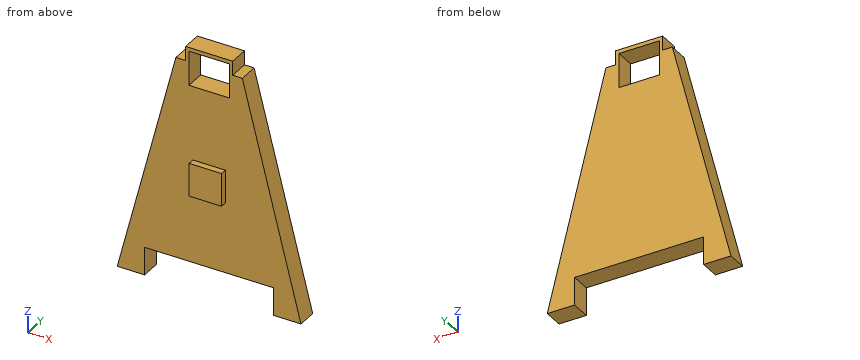
```python
from build123d import *

# Parameters (mm, degrees)
F0_W     = 1.090225624
F0_H     = 7.7231296032
F1_DEPTH = 6.35
F3_DEPTH = 8.39926


with BuildPart() as f1:
    # F0 (on Front) → F1 (new body)
    with BuildSketch(Plane.XZ):
        Polygon((-7.5686656406, 37.2254792051), (-10.668, 37.2254792051), (-29.5124314971, -36.6076258465), (-20.7240314971, -36.6076258465), (-20.7240314971, -27.6487994939), (0, -27.6487994939), (20.7240314971, -27.6487994939), (20.7240314971, -36.6076258465), (29.5124314971, -36.6076258465), (10.668, 37.2254792051), (7.5686656406, 37.2254792051), (7.5686656406, 29.5023496019), (6.4784400165, 29.5023496019), (0, 29.5023496019), (-6.4784400165, 29.5023496019), (-7.5686656406, 29.5023496019), align=None)
        with Locations((-7.0235528285, 33.3639144035)):
            Rectangle(F0_W, F0_H)
        Polygon((-7.5686656406, 41.7925901711), (-7.5686656406, 37.2254792051), (-6.4784400165, 37.2254792051), (-6.4784400165, 40.5764468014), (0, 40.5764468014), (6.4784400165, 40.5764468014), (6.4784400165, 37.2254792051), (7.5686656406, 37.2254792051), (7.5686656406, 41.7925901711), (0, 41.7925901711), align=None)
        with Locations((7.0235528285, 33.3639144035)):
            Rectangle(F0_W, F0_H)
    extrude(amount=F1_DEPTH)

    # F2 (on Front) → F3 (join)
    with BuildSketch(Plane.XZ):
        Polygon((0, 5.6396927685), (-5.2173733711, 5.6396927685), (-5.2173733711, -4.9869618379), (0, -4.9869618379), (5.2173733711, -4.9869618379), (5.2173733711, 5.6396927685), align=None)
    extrude(amount=F3_DEPTH)


solid = f1.part
```
Check sheet for the modelled part. Datum: model origin and axes. Units: mm. Round coordinates to 2 decimals unless told otherwise and drop trailing zeros. Order: outer loops, then holes, each group sorted by start corner. A loop starts at its lowest first (then second) coordinate and runs counter-clockwise, first axis right, second up. Notation, with made-up numbers: M 31,89 L 83,89 A11 ccw 83,97 Z; hole C 31.5,-26 d3. An arc over 180 degrees is marked long. Answer in a Markdown table with one row per item.
(1) Gauge pin test, flat ends, axial feed: pin 1 (12 mm diameter, centred on x = 20, z = 27, fed in from +Y); pin 2 (2 mm diameter, centred on x = -16, y = -3.5, fed in from -Z); pin 3 (3 mm diameter, centred on y = -7, z = 26, fed in from -X); pin 4 (0.9 mm diameter, centred on x = -9, y = -2, fed in from +Z). Record the tip position at first contact, or that the pin passes through.
Findings:
| item | result |
|---|---|
| pin 1 | passes through |
| pin 2 | stops at z = -27.65 |
| pin 3 | stops at x = -13.88 |
| pin 4 | stops at z = 37.23 |
(2) Section check A-A on x = 3. Record the boundary of the cut face in (y, z).
Findings:
| item | result |
|---|---|
| outline | M -8.4,-4.99 L -6.35,-4.99 L -6.35,-27.65 L 0,-27.65 L 0,29.5 L -6.35,29.5 L -6.35,5.64 L -8.4,5.64 Z; M -6.35,40.58 L 0,40.58 L 0,41.79 L -6.35,41.79 Z |
(3) Material ranges on line 1 along Z through (x, y) = (-4, -5.5); line 2 along Y through (x, z) = (2, 15.5); line 3 along Z through (x, y) = (9, -5.5), recorded low to high. Write a range as from..to.
Findings:
| item | result |
|---|---|
| line 1 | z = -27.65..29.5, 40.58..41.79 |
| line 2 | y = -6.35..0 |
| line 3 | z = -27.65..37.23 |
(4) Section check C-C on z = 36. Record the boundary of the cut face in (x, y), plus the area to 3 significant figures.
Findings:
| item | result |
|---|---|
| outline | M -10.98,-6.35 L -6.48,-6.35 L -6.48,0 L -10.98,0 Z; M 6.48,-6.35 L 10.98,-6.35 L 10.98,0 L 6.48,0 Z |
| area | 57.2 mm^2 |
(5) Section check D-D on z = 4.5. Record the boundary of the cut face in (x, y), plus the area to 3 significant figures.
Findings:
| item | result |
|---|---|
| outline | M -19.02,-6.35 L -5.22,-6.35 L -5.22,-8.4 L 5.22,-8.4 L 5.22,-6.35 L 19.02,-6.35 L 19.02,0 L -19.02,0 Z |
| area | 263 mm^2 |
(6) Section check B-B on y = -4.75. Record the boundary of the cut face in (x, z), plus the area to 3 significant figures.
Findings:
| item | result |
|---|---|
| outline | M -29.51,-36.61 L -20.72,-36.61 L -20.72,-27.65 L 20.72,-27.65 L 20.72,-36.61 L 29.51,-36.61 L 10.67,37.23 L 7.57,37.23 L 7.57,41.79 L -7.57,41.79 L -7.57,37.23 L -10.67,37.23 Z; hole M -6.48,29.5 L 6.48,29.5 L 6.48,40.58 L -6.48,40.58 Z |
| area | 2,520 mm^2 |
